from build123d import *

# Parameters (mm, degrees)
BOSS_EXTRUDE1_DEPTH = 23
FILLET1_R           = 23
SKETCH2_R           = 14
BOSS_EXTRUDE2_DEPTH = 2
HOLE1_D             = 14
FILLET2_R           = 2
FILLET3_R           = 4
RIB1_REACH          = 117.875
SKETCH5_WALL_W      = 267.881961488
SKETCH5_WALL_H      = 10
HOLE2_D             = 10


with BuildPart() as part:
    # Sketch1 → Boss-Extrude1 (new, symmetric)
    with BuildSketch(Plane.XY):
        Polygon((-87, 0), (-87, 18), (-61, 18), (-61, 14), (-32, 14), (-32, 73), (-18, 73), (-18, 14), (18, 14), (18, 73), (32, 73), (32, 14), (61, 14), (61, 18), (87, 18), (87, 0), align=None)
    extrude(amount=BOSS_EXTRUDE1_DEPTH, both=True)

    # Fillet1
    fillet1_edges = [part.edges().sort_by_distance(p)[0] for p in [
        (-25, 73, 23),
        (-25, 73, -23),
        (25, 73, -23),
        (25, 73, 23),
    ]]
    fillet(fillet1_edges, radius=FILLET1_R - 0.0001)  # a hair under: the kernel refuses the full size

    # Sketch2 → Boss-Extrude2 (add)
    with BuildSketch(Plane(origin=(-18, 0, 0), x_dir=(0, 0, -1), z_dir=(1, 0, 0))):
        with Locations(Location((0, 50, 0), (0, 0, 270))):
            Circle(SKETCH2_R)
    boss_extrude2 = extrude(amount=BOSS_EXTRUDE2_DEPTH)

    # Mirror1: Boss-Extrude2 across plane
    add(boss_extrude2.mirror(Plane(origin=(0, 0, 0), x_dir=(0, 0, 1), z_dir=(1, 0, 0))))

    # Hole1 (through all)
    with Locations(Plane(origin=(32, 0, 0), x_dir=(0, 0, -1), z_dir=(1, 0, 0))):
        with Locations((0, 50)):
            Hole(HOLE1_D / 2)

    # Fillet2
    fillet2_edges = [part.edges().sort_by_distance(p)[0] for p in [
        (-18, 64, 0),
        (18, 64, 0),
    ]]
    fillet(fillet2_edges, radius=FILLET2_R - 0.0001)  # a hair under: the kernel refuses the full size

    # Fillet3
    fillet3_edges = [part.edges().sort_by_distance(p)[0] for p in [
        (-32, 14, 0),
        (18, 14, 0),
        (61, 14, 0),
        (32, 14, 0),
        (-18, 14, 0),
        (-61, 14, 0),
    ]]
    fillet(fillet3_edges, radius=FILLET3_R - 0.0001)  # a hair under: the kernel refuses the full size

    # Sketch5 wall → Rib1 (add, up to next)
    with BuildSketch(Plane(origin=(46.5, 27, 0), x_dir=(-0.849640166198, 0.527362861778, 0), z_dir=(-0.527362861778, -0.849640166198, 0)), mode=Mode.PRIVATE) as rib1_sk1:
        Rectangle(SKETCH5_WALL_W, SKETCH5_WALL_H)
    rib1_tool1 = extrude(rib1_sk1.sketch, amount=RIB1_REACH, mode=Mode.PRIVATE) - part.part
    rib1 = rib1_tool1.solids().sort_by_distance((46.5, 27, 0))[0]
    add(rib1)

    # Mirror2: Rib1 across plane
    add(rib1.mirror(Plane(origin=(0, 0, 0), x_dir=(0, 0, 1), z_dir=(1, 0, 0))))

    # Hole2 (through all)
    with Locations(Plane(origin=(0, 18, 0), x_dir=(1, 0, 0), z_dir=(0, 1, 0))):
        with Locations((75, 12), (75, -12)):
            hole2 = Hole(HOLE2_D / 2)

    # Mirror3: Hole2 across plane
    add(hole2.mirror(Plane(origin=(0, 0, 0), x_dir=(0, 0, 1), z_dir=(1, 0, 0))), mode=Mode.SUBTRACT)


solid = part.part
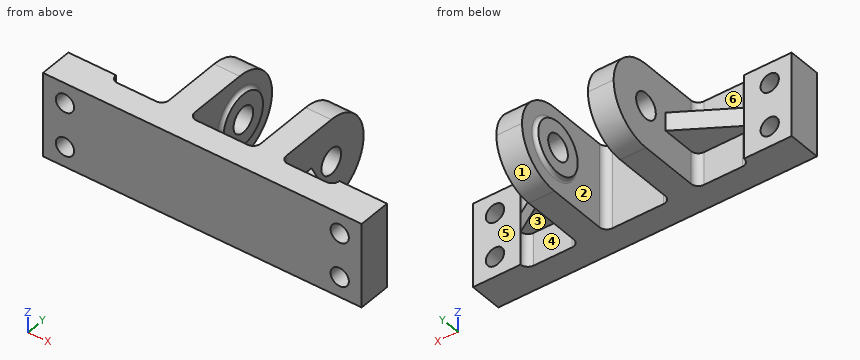
CAD build for the part. Positions are in the model's coordinates, mm. Face numbers are marked on the shaded views. A direction names the side the tool comes from. Give positions to 0.01 mm unless a question says otherwise; leave off trailing zeros. Write each loop counter-clockwise with the first axis right and the second up, starting at its lowest first coordinate (ties: lowest second). Pieces come first, ordered by that corner, then holes. Notation, with made-up numbers: M 59.5,-5 L 67.5,-5 A22 ccw 67.5,27 Z; hole C -38,-27.5 d10. An arc over 180 degrees is marked long. Put each result on its own line as item: value. Start each with the question number.
(1) Band-saw the part on C-C, the plane y = 11. Write the cut outline in (x, z).
(2) Flat gauge pins, fed straight in: pin 1 Ø5 at (y, z) = (28, 3) entering from -X; pin 2 Ø14 at (y, z) = (49.5, -0.5) entering from +X; pin 3 Ø5 at (y, z) = (59.5, -10) entering from -X. Where does each tip first touch, or does it go through?
(3) Band-saw the part on D-D, the plane x = -2. Write the cut outline in (y, z).
(4) Which spindle directions (+Z, -Z, +X, -X, +Y, -Y) get a long thin tool onto all of the face, cutting with end or side? Do the marked faces 4, 5 and 6. Say none if no direction does.
(5) Band-saw the part on B-B, the plane x = 75. Write the cut outline in (y, z), and give its area (3 significant figures).
(6) Probe L1, parallel to Y at x = 21, z = 0.5; L2, parallel to X at y = 34, z = 11; L3, parallel to Z at x = -75, y = 11. List the from-to ranges inside material, lowest first.
(7) Mould opens along Y. For the marked faces 1, 2 and 3 say: +Y half, -Y half, draft (parallel to the pull), parting line (faces both ways), or undercut.
(8) Band-saw the part on A-A, the plane y = 31.5. Write the cut outline in (x, z).
Response values:
1. outline: M -87,-23 L 87,-23 L 87,23 L -87,23 Z; hole C -75,-12 d10; hole C -75,12 d10; hole C 75,-12 d10; hole C 75,12 d10
2. pin 1: stops at x = -48.92
2. pin 2: stops at x = 32
2. pin 3: stops at x = -32
3. outline: M 0,-23 L 14,-23 L 14,23 L 0,23 Z
4. face 4: -Z, +Y
4. face 5: +Z, -Z, +X, +Y
4. face 6: +Z, +Y
5. outline: M 0,-23 L 18,-23 L 18,-17 L 0,-17 Z; M 0,-7 L 18,-7 L 18,7 L 0,7 Z; M 0,17 L 18,17 L 18,23 L 0,23 Z
5. area: 468 mm2
6. L1: y = 0 to 43.02, 56.98 to 72.99
6. L2: x = -32 to -18, 18 to 32
6. L3: z = -23 to -17, -7 to 7, 17 to 23
7. face 1: +Y half
7. face 2: undercut
7. face 3: draft
8. outline: M -39.25,-5 L -32,-5 L -32,-23 L -18,-23 L -18,23 L -32,23 L -32,5 L -39.25,5 Z; M 18,-23 L 32,-23 L 32,-5 L 39.25,-5 L 39.25,5 L 32,5 L 32,23 L 18,23 Z
